Geometry check sheet. Reference: the model listing, model coordinates, mm. Face numbers are marked on the shaded views. A direction names the side the tool comes from. Give positions to 0.01 mm unless a question says otherwise; leave off trailing zeros. Loops run counter-clockwise (first coordinate to the right, second up) from the corner with the lowest first, then second, coordinate; pieces in that order, holes last. Notation, with made-up numbers: (27, -6.75) - (55, -6.75) arc R22 ccw to (55, 17.25) - close; hole circle Ø2 at (-14, 33). An arc over 180 degrees is marked (long way). Write item = value, one per line. Start each with the question number.
from build123d import *

# Parameters (mm, degrees)
SKETCH1_R           = 12
BOSS_EXTRUDE1_DEPTH = 11.59
SKETCH3_R           = 10.5
SKETCH3_R_2         = 10
EXTRUDE_THIN1_DEPTH = 22
SHELL1_START        = -11.59
SHELL1_OUTLINE_R    = 7.5
SHELL1_DEPTH        = 18.68
CUT_EXTRUDE1_REACH  = 36.137
SKETCH4_R           = 3


# Read off the part's stored shape, not the designer's step: Shell1
with BuildPart() as part:
    # Sketch1 → Boss-Extrude1 (new, symmetric)
    with BuildSketch(Plane.XY):
        Circle(SKETCH1_R)
    extrude(amount=BOSS_EXTRUDE1_DEPTH, both=True)

    # Sketch3 → Extrude-Thin1 (add)
    with BuildSketch(Plane(origin=(0, 0, 0), x_dir=(0, 0, -1), z_dir=(1, 0, 0))):
        Circle(SKETCH3_R)
        Circle(SKETCH3_R_2, mode=Mode.SUBTRACT)
    extrude(amount=EXTRUDE_THIN1_DEPTH)

    # Shell1 outline → Shell1 (cut)
    with BuildSketch(Plane.XY.offset(SHELL1_START)):
        Circle(SHELL1_OUTLINE_R)
    extrude(amount=SHELL1_DEPTH, mode=Mode.SUBTRACT)

    # Sketch4 → Cut-Extrude1 (cut, up to next)
    with BuildSketch(Plane.XY.offset(11.59), mode=Mode.PRIVATE) as cut_extrude1_sk1:
        Circle(SKETCH4_R)
    cut_extrude1_tool1 = extrude(cut_extrude1_sk1.sketch, amount=-CUT_EXTRUDE1_REACH, mode=Mode.PRIVATE) & part.part
    add(cut_extrude1_tool1.solids().sort_by_distance((0, 0, 11.59))[0], mode=Mode.SUBTRACT)


solid = part.part
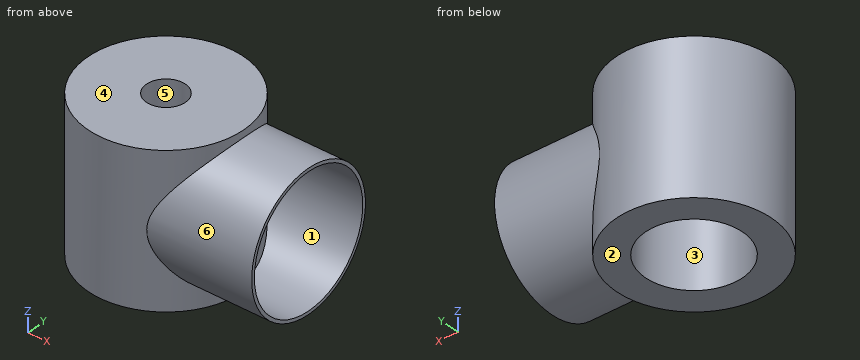
1) Cross-section at D-D on y = -7. Enter the section's corners in (x, z), and give its area (3 significant figures).
2) Cross-section at A-A on z = 0. Enter the section's corners in (x, y).
3) Material ranges on line 1 along Y through (x, z) = (0, -2.75); line 2 along Y through (x, z) = (0, 10.3); line 3 along Z through (x, y) = (12.5, 0), recorded low to high.
4) Release check for a two-part mould opening along Y. For the marked faces 4, 5 and 6 record: pulls with the +Y half, pulls with the -Y half, needs draft (parallel to the pull), parting line crosses it, or undercut.
5) Cross-section at B-B on y = 0. Enter the section's corners in (x, z), and give its area (3 significant figures).
6) Gauge pin test, flat ends, axial feed: P1, Ø3, axis at y = 0, z = 6.5, coming from the +X side; P2, Ø2, axis at x = 17, z = -3.5, coming from the -Y side; P3, Ø3, axis at x = 9, z = -0.5, coming from the -Y side. Record the tip position at first contact, or that the pin passes through.
7) Cross-section at C-C on x = 0. Enter the section's corners in (y, z).
8) Tool access check on the marked faces 1, 2 and 3. Record the directions out of +Z, -Z, +X, -X, +Y, -Y that give a thin tool (end or side, any length) a straight path to the whole face; none if there is none.
Checked values:
q1.outline = (-9.75, -11.59) - (-2.69, -11.59) - (-2.69, 7.09) - (2.69, 7.09) - (2.69, -11.59) - (9.75, -11.59) - (9.75, -7.83) - (22, -7.83) - (22, -7.14) - (9.75, -7.14) - (9.75, 7.14) - (22, 7.14) - (22, 7.83) - (9.75, 7.83) - (9.75, 11.59) - (-9.75, 11.59) - close
q1.area = 368 mm²
q2.outline = (5.81, -10.5) - (22, -10.5) - (22, -10) - (6.63, -10) arc R12 ccw to (6.63, 10) - (22, 10) - (22, 10.5) - (5.81, 10.5) arc R12 ccw (long way) to start; hole circle Ø15 at (0, 0)
q3.line_1 = -12 to -7.5, 7.5 to 12
q3.line_2 = -12 to -3, 3 to 12
q3.line_3 = -10.5 to -10, 10 to 10.5
q4.face_4 = needs draft
q4.face_5 = undercut
q4.face_6 = parting line crosses it
q5.outline = (-12, -11.59) - (-7.5, -11.59) - (-7.5, 7.09) - (-3, 7.09) - (-3, 11.59) - (-12, 11.59) - close; (3, 7.09) - (7.5, 7.09) - (7.5, -11.59) - (12, -11.59) - (12, -10.5) - (22, -10.5) - (22, -10) - (12, -10) - (12, 10) - (22, 10) - (22, 10.5) - (12, 10.5) - (12, 11.59) - (3, 11.59) - close
q5.area = 259 mm²
q6.P1 = 12
q6.P2 = -10.2
q6.P3 = -10.5
q7.outline = (-12, -11.59) - (-7.5, -11.59) - (-7.5, 7.09) - (-3, 7.09) - (-3, 11.59) - (-12, 11.59) - close; (3, 7.09) - (7.5, 7.09) - (7.5, -11.59) - (12, -11.59) - (12, 11.59) - (3, 11.59) - close
q8.face_1 = +X
q8.face_2 = -Z, +X, -X, +Y, -Y
q8.face_3 = -Z
